CAD build for the part. Positions are in the model's coordinates, mm. Face numbers are marked on the shaded views. A direction names the side the tool comes from. Give positions to 0.01 mm unless a question says otherwise; leave off trailing zeros. Loops run counter-clockwise (first coordinate to the right, second up) from the corner with the lowest first, then second, coordinate; pieces in that order, holes last. Notation, with made-up numbers: M 71,1 L 88,1 A9 cw 88,8 Z; hole C -33,30.5 d9. An arc over 180 degrees is marked long. Answer as CSV lines item,"result".
from build123d import *
from build123d.topology import SkipClean

# Parameters (mm, degrees)
SKETCH1_R           = 46.9
SKETCH1_R_2         = 36.9
BOSS_EXTRUDE1_DEPTH = 15
BOSS_EXTRUDE2_DEPTH = 20
SKETCH4_W           = 3.8
SKETCH4_H           = 13.672543204
CUT_EXTRUDE2_DEPTH  = 6
SKETCH5_R           = 1.75
CUT_EXTRUDE3_DEPTH  = 75.99479982
FILLET3_R           = 10
BOSS_EXTRUDE3_DEPTH = 15
SKETCH9_R           = 1.5
CUT_EXTRUDE4_DEPTH  = 15
CIRPATTERN1_COUNT   = 4
CUT_EXTRUDE5_DEPTH  = 15


with BuildPart() as part:
    # Sketch1 → Boss-Extrude1 (new body)
    with BuildSketch(Plane(origin=(0, 0, 0), x_dir=(1, 0, 0), z_dir=(0, 1, 0))):
        with Locations(Location((0, 0, 0), (0, 0, 270))):
            Circle(SKETCH1_R)
        with Locations(Location((0, 0, 0), (0, 0, 270))):
            Circle(SKETCH1_R_2, mode=Mode.SUBTRACT)
    extrude(amount=BOSS_EXTRUDE1_DEPTH)

    # Sketch7 → Boss-Extrude2 (add)
    with SkipClean():  # the faces are left unmerged after this step: merging them gives an invalid solid
        with BuildSketch(Plane(origin=(0, 15, 0), x_dir=(1, 0, 0), z_dir=(0, 1, 0))):
            with BuildLine():
                Line((-1.9, 46.861498055), (-1.9, 36.851051545))
                ThreePointArc((-1.9, 36.851051545), (-3.402836815, 36.742763935), (-4.9, 36.573214242))
                Line((-4.9, 36.573214242), (-4.9, 46.643327497))
                ThreePointArc((-4.9, 46.643327497), (-3.401749491, 46.776469516), (-1.9, 46.861498055))
            make_face()
            with BuildLine():
                Line((4.9, 46.643327497), (4.9, 36.573214242))
                ThreePointArc((4.9, 36.573214242), (3.402836815, 36.742763935), (1.9, 36.851051545))
                Line((1.9, 36.851051545), (1.9, 46.861498055))
                ThreePointArc((1.9, 46.861498055), (3.401749491, 46.776469516), (4.9, 46.643327497))
            make_face()
            with BuildLine():
                Line((1.9, -46.861498055), (1.9, -36.851051545))
                ThreePointArc((1.9, -36.851051545), (3.402836815, -36.742763935), (4.9, -36.573214242))
                Line((4.9, -36.573214242), (4.9, -46.643327497))
                ThreePointArc((4.9, -46.643327497), (3.401749491, -46.776469516), (1.9, -46.861498055))
            make_face()
            with BuildLine():
                Line((-4.9, -46.643327497), (-4.9, -36.573214242))
                ThreePointArc((-4.9, -36.573214242), (-3.402836815, -36.742763935), (-1.9, -36.851051545))
                Line((-1.9, -36.851051545), (-1.9, -46.861498055))
                ThreePointArc((-1.9, -46.861498055), (-3.401749491, -46.776469516), (-4.9, -46.643327497))
            make_face()
        extrude(amount=BOSS_EXTRUDE2_DEPTH)

    # Sketch4 → Cut-Extrude2 (cut)
    with SkipClean():  # the faces are left unmerged after this step: merging them gives an invalid solid
        with BuildSketch(Plane(origin=(0, 15, 0), x_dir=(1, 0, 0), z_dir=(0, 1, 0))):
            with Locations((0, 42.34115802)):
                Rectangle(SKETCH4_W, SKETCH4_H)
            with Locations((0, -42.34115802)):
                Rectangle(SKETCH4_W, SKETCH4_H)
        extrude(amount=-CUT_EXTRUDE2_DEPTH, mode=Mode.SUBTRACT)

    # Sketch5 → Cut-Extrude3 (cut, symmetric)
    with SkipClean():  # the faces are left unmerged after this step: merging them gives an invalid solid
        with BuildSketch(Plane(origin=(0, 0, 0), x_dir=(0, 0, -1), z_dir=(1, 0, 0))):
            with Locations((-41.4, 28)):
                Circle(SKETCH5_R)
        cut_extrude3 = extrude(amount=CUT_EXTRUDE3_DEPTH, both=True, mode=Mode.SUBTRACT)

    # Mirror1: Cut-Extrude3 across plane
    with SkipClean():  # the faces are left unmerged after this step: merging them gives an invalid solid
        add(cut_extrude3.mirror(Plane.XY), mode=Mode.SUBTRACT)

    # Fillet3
    # the kernel refuses this fillet: 10 mm, written as the material it adds along each edge
    with BuildSketch(Plane(origin=(-4.9, 15, -11.573214242), x_dir=(-1, 0, 0), z_dir=(0, 0, -1))) as fillet3_piece_1_section:
        with BuildLine():
            CenterArc((FILLET3_R, FILLET3_R), FILLET3_R, 180, 90)
            Line((0, FILLET3_R), (0, 0))
            Line((0, 0), (FILLET3_R, 0))
        make_face()
    fillet3_piece_1 = extrude(amount=60.070113255, mode=Mode.PRIVATE)
    fillet3_piece_1 = fillet3_piece_1 & Plane(origin=(0, 17.250849012, 0), x_dir=(0, 0, 1), z_dir=(0, -1, 0)) * Cylinder(46.9, 161, mode=Mode.PRIVATE)
    fillet3_piece_1 = fillet3_piece_1 - Plane(origin=(0, 17.250849012, 0), x_dir=(0, 0, 1), z_dir=(0, -1, 0)) * Cylinder(36.9, 161, mode=Mode.PRIVATE)
    with BuildSketch(Plane(origin=(4.9, 15, -71.643327497), x_dir=(1, 0, 0), z_dir=(0, 0, 1))) as fillet3_piece_2_section:
        with BuildLine():
            CenterArc((FILLET3_R, FILLET3_R), FILLET3_R, 180, 90)
            Line((0, FILLET3_R), (0, 0))
            Line((0, 0), (FILLET3_R, 0))
        make_face()
    fillet3_piece_2 = extrude(amount=60.070113255, mode=Mode.PRIVATE)
    fillet3_piece_2 = fillet3_piece_2 & Plane(origin=(0, 17.250856037, 0), x_dir=(0, 0, 1), z_dir=(0, -1, 0)) * Cylinder(46.9, 161, mode=Mode.PRIVATE)
    fillet3_piece_2 = fillet3_piece_2 - Plane(origin=(0, 17.250856037, 0), x_dir=(0, 0, 1), z_dir=(0, -1, 0)) * Cylinder(36.9, 161, mode=Mode.PRIVATE)
    with BuildSketch(Plane(origin=(4.9, 15, 11.573214242), x_dir=(1, 0, 0), z_dir=(0, 0, 1))) as fillet3_piece_3_section:
        with BuildLine():
            CenterArc((FILLET3_R, FILLET3_R), FILLET3_R, 180, 90)
            Line((0, FILLET3_R), (0, 0))
            Line((0, 0), (FILLET3_R, 0))
        make_face()
    fillet3_piece_3 = extrude(amount=60.070113255, mode=Mode.PRIVATE)
    fillet3_piece_3 = fillet3_piece_3 & Plane(origin=(0, 17.250849012, 0), x_dir=(0, 0, 1), z_dir=(0, -1, 0)) * Cylinder(46.9, 161, mode=Mode.PRIVATE)
    fillet3_piece_3 = fillet3_piece_3 - Plane(origin=(0, 17.250849012, 0), x_dir=(0, 0, 1), z_dir=(0, -1, 0)) * Cylinder(36.9, 161, mode=Mode.PRIVATE)
    with BuildSketch(Plane(origin=(-4.9, 15, 71.643327497), x_dir=(-1, 0, 0), z_dir=(0, 0, -1))) as fillet3_piece_4_section:
        with BuildLine():
            CenterArc((FILLET3_R, FILLET3_R), FILLET3_R, 180, 90)
            Line((0, FILLET3_R), (0, 0))
            Line((0, 0), (FILLET3_R, 0))
        make_face()
    fillet3_piece_4 = extrude(amount=60.070113255, mode=Mode.PRIVATE)
    fillet3_piece_4 = fillet3_piece_4 & Plane(origin=(0, 17.250856037, 0), x_dir=(0, 0, 1), z_dir=(0, -1, 0)) * Cylinder(46.9, 161, mode=Mode.PRIVATE)
    fillet3_piece_4 = fillet3_piece_4 - Plane(origin=(0, 17.250856037, 0), x_dir=(0, 0, 1), z_dir=(0, -1, 0)) * Cylinder(36.9, 161, mode=Mode.PRIVATE)
    add([fillet3_piece_1, fillet3_piece_2, fillet3_piece_3, fillet3_piece_4])

    # Sketch8 → Boss-Extrude3 (add)
    with BuildSketch(Plane.XZ):
        with BuildLine():
            ThreePointArc((-35.632580164, 30.494741036), (-33.163308038, 33.163308038), (-30.494741036, 35.632580164))
            Line((-30.494741036, 35.632580164), (-34.586430477, 40.027350984))
            ThreePointArc((-34.586430477, 40.027350984), (-37.405948725, 37.405948725), (-40.027350984, 34.586430477))
            Line((-40.027350984, 34.586430477), (-35.632580164, 30.494741036))
        make_face()
    boss_extrude3 = extrude(amount=-BOSS_EXTRUDE3_DEPTH)

    # Sketch9 → Cut-Extrude4 (cut)
    with BuildSketch(Plane(origin=(-37.405948725, 0, 37.405948725), x_dir=(0, -1, 0), z_dir=(-0.7071067811865488, 0, 0.7071067811865464))):
        with Locations(Location((-7.5, 0, 0), (0, 0, 90))):
            Circle(SKETCH9_R)
    cut_extrude4 = extrude(amount=-CUT_EXTRUDE4_DEPTH, mode=Mode.SUBTRACT)

    # CirPattern1: Boss-Extrude3, Cut-Extrude4 ×4 about axis
    cirpattern1_axis = Axis((0, 0, 0), (0, 1, 0))
    add([boss_extrude3.rotate(cirpattern1_axis, i * 360 / CIRPATTERN1_COUNT) for i in range(1, CIRPATTERN1_COUNT)])
    add([cut_extrude4.rotate(cirpattern1_axis, i * 360 / CIRPATTERN1_COUNT) for i in range(1, CIRPATTERN1_COUNT)], mode=Mode.SUBTRACT)

    # Sketch10 → Cut-Extrude5 (cut)
    with BuildSketch(Plane.XZ):
        with BuildLine():
            Line((-35.632580164, 30.494741036), (-31.833797631, 27.243702546))
            ThreePointArc((-31.833797631, 27.243702546), (-41.9, 0), (-31.833797631, -27.243702546))
            Line((-31.833797631, -27.243702546), (-35.632580164, -30.494741036))
            ThreePointArc((-35.632580164, -30.494741036), (-46.9, 0), (-35.632580164, 30.494741036))
        make_face()
        with BuildLine():
            Line((35.632580164, -30.494741036), (31.833797631, -27.243702546))
            ThreePointArc((31.833797631, -27.243702546), (41.9, 0), (31.833797631, 27.243702546))
            Line((31.833797631, 27.243702546), (35.632580164, 30.494741036))
            ThreePointArc((35.632580164, 30.494741036), (46.9, 0), (35.632580164, -30.494741036))
        make_face()
    extrude(amount=-CUT_EXTRUDE5_DEPTH, mode=Mode.SUBTRACT)


solid = part.part
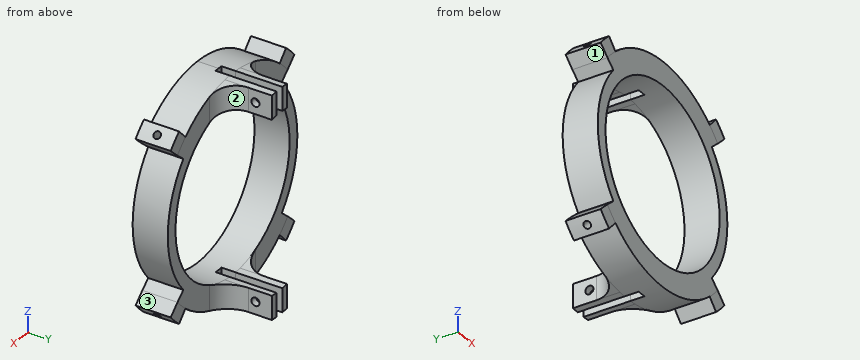
1) Band-saw the part on A-A on z = 0. Give the cut face in (x, y), and give its area (3 significant figures).
Answer below:
outline,"M -41.9,0 L -36.9,0 L -36.9,15 L -41.9,15 Z; M 36.9,0 L 41.9,0 L 41.9,15 L 36.9,15 Z"
area,"150 mm^2"
2) Band-saw the part on C-C on y = 21. Give the cut face in (x, z), and give its area (3 significant figures).
Answer below:
outline,"M -5.73,-46.55 A46.9 ccw -1.9,-46.86 L -1.9,-36.85 A36.9 cw -5.73,-36.45 Z; M -5.73,36.45 A36.9 cw -1.9,36.85 L -1.9,46.86 A46.9 ccw -5.73,46.55 Z; M 1.9,-46.86 A46.9 ccw 5.73,-46.55 L 5.73,-36.45 A36.9 cw 1.9,-36.85 Z; M 1.9,36.85 A36.9 cw 5.73,36.45 L 5.73,46.55 A46.9 ccw 1.9,46.86 Z"
area,"154 mm^2"
3) Drill centre lines: line 1 (X direction, y = 26, z = 37.5); line 2 (Z direction, x = -5, y = 12.5); line 3 (Y direction, x = -3.65, z = 41.4). Where is each one in solid material? Low to high. Write a range as from..to.
Answer below:
line 1,"x = -4.9..-1.9, 1.9..4.9"
line 2,"z = -46.63..-36.56, 36.56..46.63"
line 3,"y = 0..26.25, 29.75..35"
4) Band-saw the part on B-B on y = 28. Give the number of separate pieces and of enclosed holes in the cut face, and give its area (3 significant figures).
Answer below:
separate pieces,"8"
enclosed holes,"0"
area,"78.4 mm^2"
5) Flat gauge pins, fed straight in: pin 1 (3 mm diameter, centred on y = 32.5, z = 40.5, fed in from -X); pin 2 (10.5 mm diameter, centred on x = -33.5, z = -35.5, fed in from +Y); pin 3 (2 mm diameter, centred on y = 28, z = 41.4, fed in from -X); pin 4 (3 mm diameter, centred on y = 27.5, z = 42.5, fed in from +X). Where does each tip first touch, or does it go through?
Answer below:
pin 1,"stops at x = -4.9"
pin 2,"stops at y = 15"
pin 3,"passes through"
pin 4,"stops at x = 4.9"
6) Which spindle directions (+Z, -Z, +X, -X, +Y, -Y) get a long thin tool onto all of the face, cutting with end or side? Do the marked faces 1, 2 and 3. Say none if no direction does.
Answer below:
face 1,"-X, +Y, -Y"
face 2,"+Z, -Z, +X, +Y"
face 3,"+X, +Y, -Y"
